Part model, mm, in its own coordinate system. Face numbers are marked on the shaded views. Coordinates: 2 decimals unless noted, no trailing zeros. Order: outer loops, then holes, each group sorted by start corner. A loop starts at its lowest first (then second) coordinate and runs counter-clockwise, first axis right, second up.
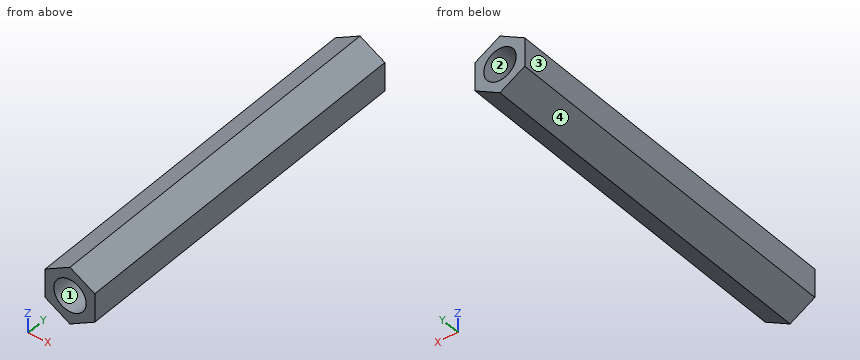
Autodesk Inventor part; units mm, degrees
ref_plane "YZ Plane" through (0, 0, 0) normal (1, 0, 0) x (0, 1, 0)
ref_plane "XZ Plane" through (0, 0, 0) normal (0, 1, 0) x (-1, 0, 0)
ref_plane "XY Plane" through (0, 0, 0) normal (0, 0, 1) x (1, 0, 0)
sketch "Sketch1" plane through (0, 0, 0) normal (0, 1, 0) x (-1, 0, 0)
  line L0 (0, -2.6558) -> (-2.3, -1.3279)
  line L1 (-2.3, -1.3279) -> (-2.3, 1.3279)
  line L2 (-2.3, 1.3279) -> (0, 2.6558)
  line L3 (0, 2.6558) -> (2.3, 1.3279)
  line L4 (2.3, 1.3279) -> (2.3, -1.3279)
  line L5 (2.3, -1.3279) -> (0, -2.6558)
  point P0 (0, 0)
  point P1 (0, 0)
  dimension "d0" = 4.6
extrude "Extrusion1" add sketch "Sketch1" along normal blind 34
sketch "Sketch2" plane through (0, 34, 0) normal (0, 1, 0) x (1, 0, 0)
  circle A0 centre (0, 0) radius 1.5
  dimension "d3" = 3
extrude "Extrusion2" cut sketch "Sketch2" against normal blind 10
sketch "Sketch3" plane through (0, 0, 0) normal (0, -1, 0) x (1, 0, 0)
  circle A0 centre (0, 0) radius 1.5
  dimension "d6" = 3
extrude "Extrusion3" cut sketch "Sketch3" against normal blind 10
properties part number "M3_34_MM_STANDOFF_PIN"
Q1. Pin check, flat tips, straight feed: pin 1 Ø0.9 at (x, z) = (-0.5, 0.5) entering from +Y; pin 2 Ø1.5 at (x, z) = (0, -0.5) entering from -Y. Stop position of each tip, or through.
Results list:
pin 1: stops at y = 24
pin 2: stops at y = 10
Q2. Wall check: line 1 along X through (y, z) = (28.5, 0); line 2 along Y through (x, z) = (-1, -0.75); line 3 along X through (y, z) = (30, -0.5). Give the ranges that are in metal, low to high.
Results list:
line 1: x = -2.3 to -1.5, 1.5 to 2.3
line 2: y = 10 to 24
line 3: x = -2.3 to -1.41, 1.41 to 2.3
Q3. Cut at B-B on z = 0. Write the cut outline in (x, y).
Results list:
outline: (-2.3, 0) - (-1.5, 0) - (-1.5, 10) - (1.5, 10) - (1.5, 0) - (2.3, 0) - (2.3, 34) - (1.5, 34) - (1.5, 24) - (-1.5, 24) - (-1.5, 34) - (-2.3, 34) - close
Q4. Mould opens along Z. For the marked faces 1, 2, 3 and 4 say: pulls with the +Z half, pulls with the -Z half, needs draft (parallel to the pull), parting line crosses it, or undercut.
Results list:
face 1: undercut
face 2: undercut
face 3: needs draft
face 4: pulls with the -Z half
Q5. Cut at C-C on x = 0.6. Write the cut outline in (y, z).
Results list:
outline: (0, -2.31) - (34, -2.31) - (34, -1.37) - (24, -1.37) - (24, 1.37) - (34, 1.37) - (34, 2.31) - (0, 2.31) - (0, 1.37) - (10, 1.37) - (10, -1.37) - (0, -1.37) - close
Q6. Cut at A-A on y = 3. Write the cut outline in (x, z), and give its area (3 significant figures).
Results list:
outline: (-2.3, -1.33) - (0, -2.66) - (2.3, -1.33) - (2.3, 1.33) - (0, 2.66) - (-2.3, 1.33) - close; hole circle Ø3 at (0, 0)
area: 11.3 mm2
Q7. Cut at D-D on y = 20. Write the cut outline in (x, z), and give its area (3 significant figures).
Results list:
outline: (-2.3, -1.33) - (0, -2.66) - (2.3, -1.33) - (2.3, 1.33) - (0, 2.66) - (-2.3, 1.33) - close
area: 18.3 mm2
